Check sheet for the modelled part. Datum: model origin and axes. Units: mm. Face numbers are marked on the shaded views. Round coordinates to 2 decimals unless told otherwise and drop trailing zeros. Loops run counter-clockwise (first coordinate to the right, second up) from the corner with the lowest first, then second, coordinate; pieces in that order, holes last. Notation, with made-up numbers: (-28, 44.25) - (-15, 44.25) arc R25 ccw to (-15, 56.25) - close; hole circle Ø8 at (72.5, 1.5). An arc over 180 degrees is marked (long way). Put each result on its own line as item: value.
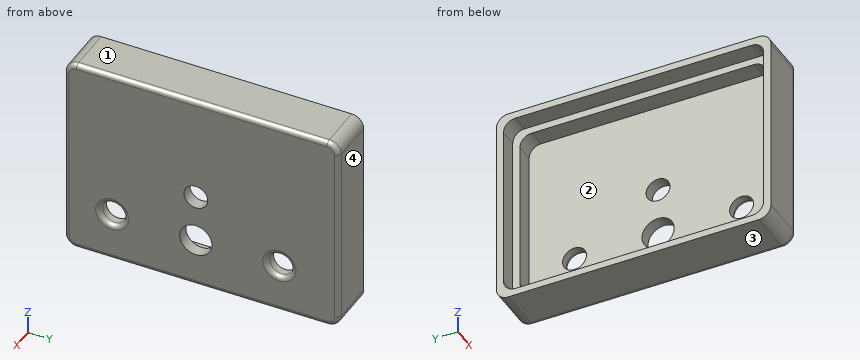
```python
from build123d import *

# Parameters (mm, degrees)
SKETCH1_W           = 43.18
SKETCH1_H           = 58.42
BOSS_EXTRUDE1_DEPTH = 10.16
SKETCH2_R           = 2.54
SKETCH2_R_2         = 3.429
CUT_EXTRUDE2_DEPTH  = 66.806860754
SKETCH3_W           = 37.132
SKETCH3_H           = 52.324
CUT_EXTRUDE3_DEPTH  = 7.62
SKETCH4_W           = 40.18
SKETCH4_H           = 55.372
CUT_EXTRUDE4_DEPTH  = 3.81
FILLET1_R           = 2.54
FILLET2_R           = 2.54
FILLET3_R           = 2.54
FILLET4_R           = 2.54
FILLET5_R           = 2.54
FILLET6_R           = 1
FILLET7_R           = 1
FILLET8_R           = 1


with BuildPart() as part:
    # Sketch1 → Boss-Extrude1 (new body)
    with BuildSketch(Plane(origin=(0, 0, 0), x_dir=(0, 0, -1), z_dir=(1, 0, 0))):
        with Locations((6.948060942, 29.21)):
            Rectangle(SKETCH1_W, SKETCH1_H)
    extrude(amount=BOSS_EXTRUDE1_DEPTH)

    # Sketch2 → Cut-Extrude2 (cut, through all)
    with BuildSketch(Plane.ZY):
        with Locations((-17.960793947, 10.16)):
            Circle(SKETCH2_R)
        with Locations((-17.960793947, 45.72)):
            Circle(SKETCH2_R)
        with Locations((-17.960793947, 27.94)):
            Circle(SKETCH2_R_2)
        with Locations((-7.800793947, 27.94)):
            Circle(SKETCH2_R)
    extrude(amount=-CUT_EXTRUDE2_DEPTH, mode=Mode.SUBTRACT)

    # Sketch3 → Cut-Extrude3 (cut)
    with BuildSketch(Plane.ZY):
        with Locations((-6.972060942, 29.21)):
            Rectangle(SKETCH3_W, SKETCH3_H)
    extrude(amount=-CUT_EXTRUDE3_DEPTH, mode=Mode.SUBTRACT)

    # Sketch4 → Cut-Extrude4 (cut)
    with BuildSketch(Plane.ZY):
        with Locations((-6.972060942, 29.21)):
            Rectangle(SKETCH4_W, SKETCH4_H)
    extrude(amount=-CUT_EXTRUDE4_DEPTH, mode=Mode.SUBTRACT)

    # Fillet1
    fillet1_edges = [part.edges().sort_by_distance(p)[0] for p in [
        (5.715, 3.048, -25.538060942),
        (1.905, 1.524, -27.062060942),
    ]]
    fillet(fillet1_edges, radius=FILLET1_R)

    # Fillet2
    fillet2_edges = [part.edges().sort_by_distance(p)[0] for p in [
        (5.715, 3.048, 11.593939058),
        (1.905, 1.524, 13.117939058),
    ]]
    fillet(fillet2_edges, radius=FILLET2_R)

    # Fillet3
    fillet3_edges = [part.edges().sort_by_distance(p)[0] for p in [
        (5.715, 55.372, 11.593939058),
        (1.905, 56.896, 13.117939058),
    ]]
    fillet(fillet3_edges, radius=FILLET3_R)

    # Fillet4
    fillet4_edges = [part.edges().sort_by_distance(p)[0] for p in [
        (5.715, 55.372, -25.538060942),
        (1.905, 56.896, -27.062060942),
    ]]
    fillet(fillet4_edges, radius=FILLET4_R)

    # Fillet5
    fillet5_edges = [part.edges().sort_by_distance(p)[0] for p in [
        (5.08, 58.42, 14.641939058),
        (5.08, 58.42, -28.538060942),
        (5.08, 0, -28.538060942),
        (5.08, 0, 14.641939058),
    ]]
    fillet(fillet5_edges, radius=FILLET5_R)

    # Fillet6
    fillet6_edges = [part.edges().sort_by_distance(p)[0] for p in [
        (10.16, 29.21, -28.538060942),
        (10.16, 0, -6.948060942),
        (10.16, 29.21, 14.641939058),
        (10.16, 58.42, -6.948060942),
        (10.16, 57.676051224, 13.897990282),
        (10.16, 57.676051224, -27.794112166),
        (10.16, 0.743948776, 13.897990282),
        (10.16, 0.743948776, -27.794112166),
    ]]
    fillet(fillet6_edges, radius=FILLET6_R)

    # Fillet7
    fillet7_edges = [part.edges().sort_by_distance(p)[0] for p in [
        (10.16, 45.72, -20.500793947),
    ]]
    fillet(fillet7_edges, radius=FILLET7_R)

    # Fillet8
    fillet8_edges = [part.edges().sort_by_distance(p)[0] for p in [
        (10.16, 10.16, -20.500793947),
    ]]
    fillet(fillet8_edges, radius=FILLET8_R)


solid = part.part
```
Item 1: Release check for a two-part mould opening along Z. For the marked faces 1, 2, 3 and 4 record: +Z half, -Z half, draft (parallel to the pull), parting line (faces both ways), or undercut.
Filled sheet:
face 1: +Z half
face 2: undercut
face 3: -Z half
face 4: draft
Item 2: Section check D-D on z = 2. Enter the section's corners in (x, y), then the cut area to 3 significant figures.
Filled sheet:
outline: (0, 0) - (9.16, 0) arc R1 ccw to (10.16, 1) - (10.16, 57.42) arc R1 ccw to (9.16, 58.42) - (0, 58.42) - (0, 56.9) - (3.81, 56.9) - (3.81, 55.37) - (7.62, 55.37) - (7.62, 3.05) - (3.81, 3.05) - (3.81, 1.52) - (0, 1.52) - close
area: 183 mm²
Item 3: Section check B-B on y = 27.94. Enter the section's corners in (x, z).
Filled sheet:
outline: (0, -28.54) - (9.16, -28.54) arc R1 ccw to (10.16, -27.54) - (10.16, -21.39) - (7.62, -21.39) - (7.62, -25.54) - (3.81, -25.54) - (3.81, -27.06) - (0, -27.06) - close; (0, 13.12) - (3.81, 13.12) - (3.81, 11.59) - (7.62, 11.59) - (7.62, -5.26) - (10.16, -5.26) - (10.16, 13.64) arc R1 ccw to (9.16, 14.64) - (0, 14.64) - close; (7.62, -14.53) - (10.16, -14.53) - (10.16, -10.34) - (7.62, -10.34) - close
Item 4: Section check A-A on x = 4.75. Enter the section's corners in (y, z), then the cut area to 3 significant figures.
Filled sheet:
outline: (0, -26) arc R2.54 ccw to (2.54, -28.54) - (55.88, -28.54) arc R2.54 ccw to (58.42, -26) - (58.42, 12.1) arc R2.54 ccw to (55.88, 14.64) - (2.54, 14.64) arc R2.54 ccw to (0, 12.1) - close; hole (3.05, -23) arc R2.54 ccw to (5.59, -25.54) - (52.83, -25.54) arc R2.54 ccw to (55.37, -23) - (55.37, 9.05) arc R2.54 ccw to (52.83, 11.59) - (5.59, 11.59) arc R2.54 ccw to (3.05, 9.05) - close
area: 580 mm²
Item 5: Section check C-C on y = 45.72. Enter the section's corners in (x, z).
Filled sheet:
outline: (0, -28.54) - (9.16, -28.54) arc R1 ccw to (10.16, -27.54) - (10.16, -21.5) arc R1 ccw to (9.16, -20.5) - (7.62, -20.5) - (7.62, -25.54) - (3.81, -25.54) - (3.81, -27.06) - (0, -27.06) - close; (0, 13.12) - (3.81, 13.12) - (3.81, 11.59) - (7.62, 11.59) - (7.62, -15.42) - (9.16, -15.42) arc R1 ccw to (10.16, -14.42) - (10.16, 13.64) arc R1 ccw to (9.16, 14.64) - (0, 14.64) - close
Item 6: Thickness scan on line 1 (Y direction, x = 1.5, z = -6); line 2 (Y direction, x = 7, z = -13); line 3 (Z direction, x = 1, y = 40). Record the ranges inside material, lowest first. Write a range as from..to.
Filled sheet:
line 1: 0..1.52, 56.9..58.42
line 2: 0..3.05, 55.37..58.42
line 3: -28.54..-27.06, 13.12..14.64
Item 7: Go/stop test with flat-tipped pins: pin 1 (2 mm diameter, centred on y = 38, z = 2, fed in from -X); pin 2 (6.5 mm diameter, centred on y = 10.16, z = -17.96, fed in from +X). Record where each tip stops, or that it passes through.
Filled sheet:
pin 1: x = 7.62
pin 2: x = 10.12
